Input: part model. Units: mm. Frame: model coordinates. A direction names the side the tool comes from. Round coordinates to 2 decimals unless told otherwise and drop trailing zeros. Loops run counter-clockwise (first coordinate to the right, second up) from the corner with the lowest first, then second, coordinate; pieces in that order, holes last.
1) Section C-C, the plane y = -0.5. Return loops of the section in (x, z) (3 decimals), and give its area (3 significant figures).
2) Section D-D, the plane x = -0.25. Return loops of the section in (y, z).
3) Section A-A, the plane x = 3.25. Return loops of the section in (y, z).
4) Draft query along X for faces 3 (the face through (6.175, 0, -1)), 4 (the face through (-4.275, 0, -1)), 5 (the face through (0, 0, 2.898)). Return one class per face: pulls with the +X half, pulls with the -X half, needs draft (parallel to the pull), parting line crosses it, or undercut.
5) Ray query, line 1 along X through (y, z) = (3, -1.75) (3 decimals); line 2 along Z through (x, y) = (4, -5); line 3 along Z through (x, y) = (0, -4.25). Return the intervals inside material, ascending.
6) First-contact query: pin 1 (1.5 mm diameter, centred on x = -0.5, y = -3, fed in from -Z). Flat tip, straight axial feed; report the tip coordinate or a pass-through.
7) Section B-B, the plane z = -2.5. Return loops of the section in (x, y) (3 decimals).
8) Access query for faces 1 (the face through (-4, 0, -4.552)), 2 (the face through (0, 0, 1.898)). Directions: +Z, -Z, +X, -X, +Y, -Y. A direction counts if a zero-diameter tool reaches every point of the face in a straight line with its end or side. Return the directions, or none.
from build123d import *

# Parameters (mm, degrees)
F1_DEPTH = 6
F2_R     = 0.5
F3_R     = 0.5


with BuildPart() as f1:
    # F0 (on Front) → F1 (new body, symmetric)
    with BuildSketch(Plane.XZ):
        Polygon((6.175, -4.5523648744), (6.175, 2.8976351256), (-6.175, 2.8976351256), (-6.175, -4.5523648744), (-2.2, -4.5523648744), (-2.2, -3.3523648744), (-4.275, -3.3523648744), (-4.275, 1.8976351256), (4.275, 1.8976351256), (4.275, -3.3523648744), (2.2, -3.3523648744), (2.2, -4.5523648744), align=None)
    extrude(amount=F1_DEPTH, both=True)

    # F2
    f2_edges = [f1.edges().sort_by_distance(p)[0] for p in [
        (-2.2, 0, -4.552365),
        (2.2, 0, -4.552365),
        (-2.2, 0, -3.352365),
        (2.2, 0, -3.352365),
    ]]
    fillet(f2_edges, radius=F2_R)

    # F3
    f3_edges = [f1.edges().sort_by_distance(p)[0] for p in [
        (6.175, 0, -4.552365),
        (6.175, 6, -0.827365),
        (6.175, 0, 2.897635),
        (6.175, -6, -0.827365),
        (0, 6, 2.897635),
        (-6.175, 0, 2.897635),
        (0, -6, 2.897635),
        (-6.175, 6, -0.827365),
        (-6.175, 0, -4.552365),
        (-6.175, -6, -0.827365),
    ]]
    fillet(f3_edges, radius=F3_R)


solid = f1.part
Final values:
1. outline: (-6.175, -4.052) arc R0.5 ccw to (-5.675, -4.552) - (-2.7, -4.552) arc R0.5 ccw to (-2.2, -4.052) - (-2.2, -3.852) arc R0.5 ccw to (-2.7, -3.352) - (-4.275, -3.352) - (-4.275, 1.898) - (4.275, 1.898) - (4.275, -3.352) - (2.7, -3.352) arc R0.5 ccw to (2.2, -3.852) - (2.2, -4.052) arc R0.5 ccw to (2.7, -4.552) - (5.675, -4.552) arc R0.5 ccw to (6.175, -4.052) - (6.175, 2.398) arc R0.5 ccw to (5.675, 2.898) - (-5.675, 2.898) arc R0.5 ccw to (-6.175, 2.398) - close
1. area: 41.4 mm2
2. outline: (-6, 1.9) - (6, 1.9) - (6, 2.4) arc R0.5 ccw to (5.5, 2.9) - (-5.5, 2.9) arc R0.5 ccw to (-6, 2.4) - close
3. outline: (-6, -4.55) - (6, -4.55) - (6, -3.35) - (-6, -3.35) - close; (-6, 1.9) - (6, 1.9) - (6, 2.4) arc R0.5 ccw to (5.5, 2.9) - (-5.5, 2.9) arc R0.5 ccw to (-6, 2.4) - close
4. face 3: pulls with the +X half
4. face 4: undercut
4. face 5: needs draft
5. line 1: x = -6.175 to -4.275, 4.275 to 6.175
5. line 2: z = -4.55 to -3.35, 1.9 to 2.9
5. line 3: z = 1.9 to 2.9
6. pin 1: stops at z = 1.9
7. outline: (-6.175, -5.5) arc R0.5 ccw to (-5.675, -6) - (-4.275, -6) - (-4.275, 6) - (-5.675, 6) arc R0.5 ccw to (-6.175, 5.5) - close; (4.275, -6) - (5.675, -6) arc R0.5 ccw to (6.175, -5.5) - (6.175, 5.5) arc R0.5 ccw to (5.675, 6) - (4.275, 6) - close
8. face 1: -Z, +X, -X, +Y, -Y
8. face 2: +Y, -Y
